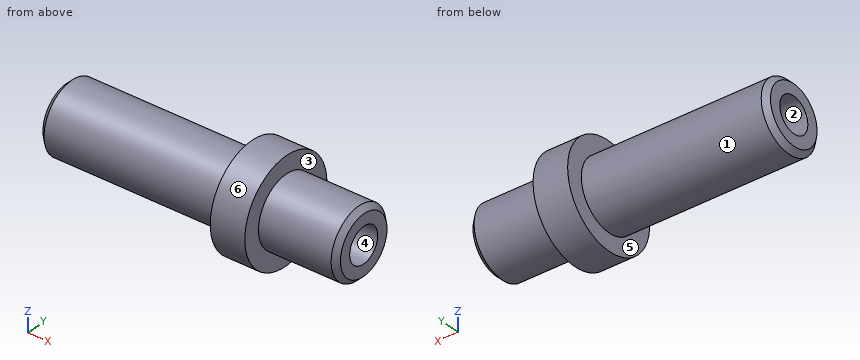
```python
from build123d import *

# Parameters (mm, degrees)
TROU_TARAUD_M2_51_D     = 2.05
TROU_TARAUD_M2_51_DEPTH = 8
TROU_TARAUD_M2_51_TIP   = 0.615882135
TROU_TARAUD_M2_52_D     = 2.05
TROU_TARAUD_M2_52_DEPTH = 8
TROU_TARAUD_M2_52_TIP   = 0.615882135
CHANFREIN1_SIZE         = 0.3


with BuildPart() as part:
    # Esquisse1 → Révolution1 (revolve)
    with BuildSketch(Plane.XY):
        Polygon((0, 0), (0, 2), (10.7, 2), (10.7, 3), (12.7, 3), (12.7, 2), (17.2, 2), (17.2, 0), align=None)
    revolve(axis=Axis((17.2, 0, 0), (-1, 0, 0)))

    # Trou taraudé M2.51
    with Locations(Plane.ZY):
        with Locations((0, 0)):
            Hole(TROU_TARAUD_M2_51_D / 2, depth=TROU_TARAUD_M2_51_DEPTH)
            with Locations((0, 0, -(TROU_TARAUD_M2_51_DEPTH + TROU_TARAUD_M2_51_TIP / 2))):  # 118° drill point
                Cone(0, TROU_TARAUD_M2_51_D / 2, TROU_TARAUD_M2_51_TIP, mode=Mode.SUBTRACT)

    # Trou taraudé M2.52
    with Locations(Plane(origin=(17.2, 0, 0), x_dir=(0, 0, -1), z_dir=(1, 0, 0))):
        with Locations((0, 0)):
            Hole(TROU_TARAUD_M2_52_D / 2, depth=TROU_TARAUD_M2_52_DEPTH)
            with Locations((0, 0, -(TROU_TARAUD_M2_52_DEPTH + TROU_TARAUD_M2_52_TIP / 2))):  # 118° drill point
                Cone(0, TROU_TARAUD_M2_52_D / 2, TROU_TARAUD_M2_52_TIP, mode=Mode.SUBTRACT)

    # Chanfrein1
    chanfrein1_edges = [part.edges().sort_by_distance(p)[0] for p in [
        (17.2, -2, 0),
        (0, -2, 0),
    ]]
    chamfer(chanfrein1_edges, length=CHANFREIN1_SIZE)


solid = part.part
```
Geometry check sheet. Reference: the model listing, model coordinates, mm. Face numbers are marked on the shaded views. A direction names the side the tool comes from. Give positions to 0.01 mm unless a question says otherwise; leave off trailing zeros. Order: outer loops, then holes, each group sorted by start corner. A loop starts at its lowest first (then second) coordinate and runs counter-clockwise, first axis right, second up. Notation, with made-up numbers: (78.25, -37.5) - (84.25, -37.5) arc R8 cw to (84.25, -25.5) - close; hole circle Ø2 at (18.25, -31). An arc over 180 degrees is marked (long way). Answer in a Markdown table with one row per item. Add a question column.
Q1. Mould release check, pull along Y, two halves, no side actions. Record for the marked faces 1, 2 and 3: pulls with the +Y half, pulls with the -Y half, needs draft (parallel to the pull), parting line crosses it, or undercut.
Q2. Cross-section at D-D, the plane x = 9. Enter the section's corners in (y, z), then the cut area to 3 significant figures.
Q3. Gauge pin test, flat ends, axial feed: pin 1 (3 mm diameter, centred on x = 11, y = 2, fed in from -Z); pin 2 (1.5 mm diameter, centred on x = 14.5, y = 0.5, fed in from -Z); pin 3 (1.5 mm diameter, centred on y = -2, z = -1.5, fed in from -X). Record the tip position at first contact, or that the pin passes through.
Q4. Cross-section at C-C, the plane z = 2.5. Enter the section's corners in (x, y).
Q5. Tool access check on the marked faces 4, 5 and 6. Record the directions out of +Z, -Z, +X, -X, +Y, -Y that give a thin tool (end or side, any length) a straight path to the whole face; none if there is none.
Q6. Cross-section at B-B, the plane y = 2.35. Enter the section's corners in (x, z).
Q7. Material ranges on probe 1 along Y at (x, z) = (14.75, 0) (3 decimals); probe 2 along Y at (x, z) = (11.5, 0) (3 decimals), recorded low to high. Write a range as from..to.
Q8. Cross-section at A-A, the plane x = 12.5. Enter the section's corners in (y, z) (3 decimals), then the cut area to 3 significant figures.
Check values:
| question | item | result |
|---|---|---|
| 1 | face 1 | parting line crosses it |
| 1 | face 2 | undercut |
| 1 | face 3 | needs draft |
| 2 | outline | circle Ø4 at (0, 0); hole circle Ø1.38 at (0, 0) |
| 2 | area | 11.1 mm^2 |
| 3 | pin 1 | stops at z = -2.96 |
| 3 | pin 2 | stops at z = -2 |
| 3 | pin 3 | stops at x = 0.05 |
| 4 | outline | (10.7, -1.66) - (12.7, -1.66) - (12.7, 1.66) - (10.7, 1.66) - close |
| 5 | face 4 | +X |
| 5 | face 5 | -X |
| 5 | face 6 | +X, -X |
| 6 | outline | (10.7, -1.86) - (12.7, -1.86) - (12.7, 1.86) - (10.7, 1.86) - close |
| 7 | probe 1 | y = -2..-1.025, 1.025..2 |
| 7 | probe 2 | y = -3..-1.025, 1.025..3 |
| 8 | outline | circle Ø6 at (0, 0); hole circle Ø2.05 at (0, 0) |
| 8 | area | 25.0 mm^2 |
